from build123d import *

# Parameters (mm, degrees)
SKETCH1_W           = 45.2
SKETCH1_H           = 20.6
BOSS_EXTRUDE1_DEPTH = 1.1
SKETCH18_R          = 1
CUT_EXTRUDE4_DEPTH  = 25.860812537


with BuildPart() as part:
    # Sketch1 → Boss-Extrude1 (new body)
    with BuildSketch(Plane(origin=(0, 0, 0), x_dir=(1, 0, 0), z_dir=(0, 1, 0))):
        Rectangle(SKETCH1_W, SKETCH1_H)
    extrude(amount=BOSS_EXTRUDE1_DEPTH)

    # Sketch18 → Cut-Extrude4 (cut, through all)
    with BuildSketch(Plane(origin=(0, 1.1, 0), x_dir=(1, 0, 0), z_dir=(0, 1, 0))):
        with Locations(Location((-21.2, -8.9, 0), (0, 0, 270))):
            Circle(SKETCH18_R)
        with Locations(Location((21.2, 8.9, 0), (0, 0, 270))):
            Circle(SKETCH18_R)
    cut_extrude4 = extrude(amount=-CUT_EXTRUDE4_DEPTH, mode=Mode.SUBTRACT)

    # Mirror1: Cut-Extrude4 across plane
    add(cut_extrude4.mirror(Plane(origin=(0, 0, 0), x_dir=(0, 0, 1), z_dir=(1, 0, 0))), mode=Mode.SUBTRACT)


solid = part.part
The model under review builds one solid part; all positions refer to its coordinate system, in mm. Coordinates: 2 decimals unless noted, no trailing zeros. Order: outer loops, then holes, each group sorted by start corner. A loop starts at its lowest first (then second) coordinate and runs counter-clockwise, first axis right, second up. Notation, with made-up numbers: (29.25, 56) -> (79.25, 56) arc R23 ccw to (79.25, 66) -> close; hole circle Ø11 at (77, 8.25). An arc over 180 degrees is marked (long way). Answer in a Markdown table with one row per item.
(1) Consider section A-A (z = -8.9). Write out the cut boundary in (x, y), plus the area to 3 significant figures.
Answers:
| item | result |
|---|---|
| outline | (-22.6, 0) -> (-22.2, 0) -> (-22.2, 1.1) -> (-22.6, 1.1) -> close; (-20.2, 0) -> (20.2, 0) -> (20.2, 1.1) -> (-20.2, 1.1) -> close; (22.2, 0) -> (22.6, 0) -> (22.6, 1.1) -> (22.2, 1.1) -> close |
| area | 45.3 mm² |
(2) Wall thickness on line 1 along X through (y, z) = (0.55, 8.9): over which ranges is the line inside the solid? List them lowest first.
Answers:
| item | result |
|---|---|
| line 1 | -22.6 to -22.2, -20.2 to 20.2, 22.2 to 22.6 |
(3) The part is to be moulded in two halves that separate along Z. For faces 1 (the cylindrical face through (-21.8, 0.6, 8.1)), 2 (the flat face through (-0.3, 0.5, 10.3)), 3 (the flat face through (0, 1.1, 0)), say which applies: +Z half, -Z half, draft (parallel to the pull), parting line (faces both ways), or undercut.
Answers:
| item | result |
|---|---|
| face 1 | undercut |
| face 2 | +Z half |
| face 3 | draft |
(4) Consider section B-B (x = -21.2). Write out the cut boundary in (y, z).
Answers:
| item | result |
|---|---|
| outline | (0, -10.3) -> (1.1, -10.3) -> (1.1, -9.9) -> (0, -9.9) -> close; (0, -7.9) -> (1.1, -7.9) -> (1.1, 7.9) -> (0, 7.9) -> close; (0, 9.9) -> (1.1, 9.9) -> (1.1, 10.3) -> (0, 10.3) -> close |
(5) Insertion check: pin 1 (1.6 mm diameter, centred on x = -21.2, z = -8.9, fed in from -Y). The pin has a flat end and moves straight along its axis. Give the tip position at first contact, or say it passes through.
Answers:
| item | result |
|---|---|
| pin 1 | through |
